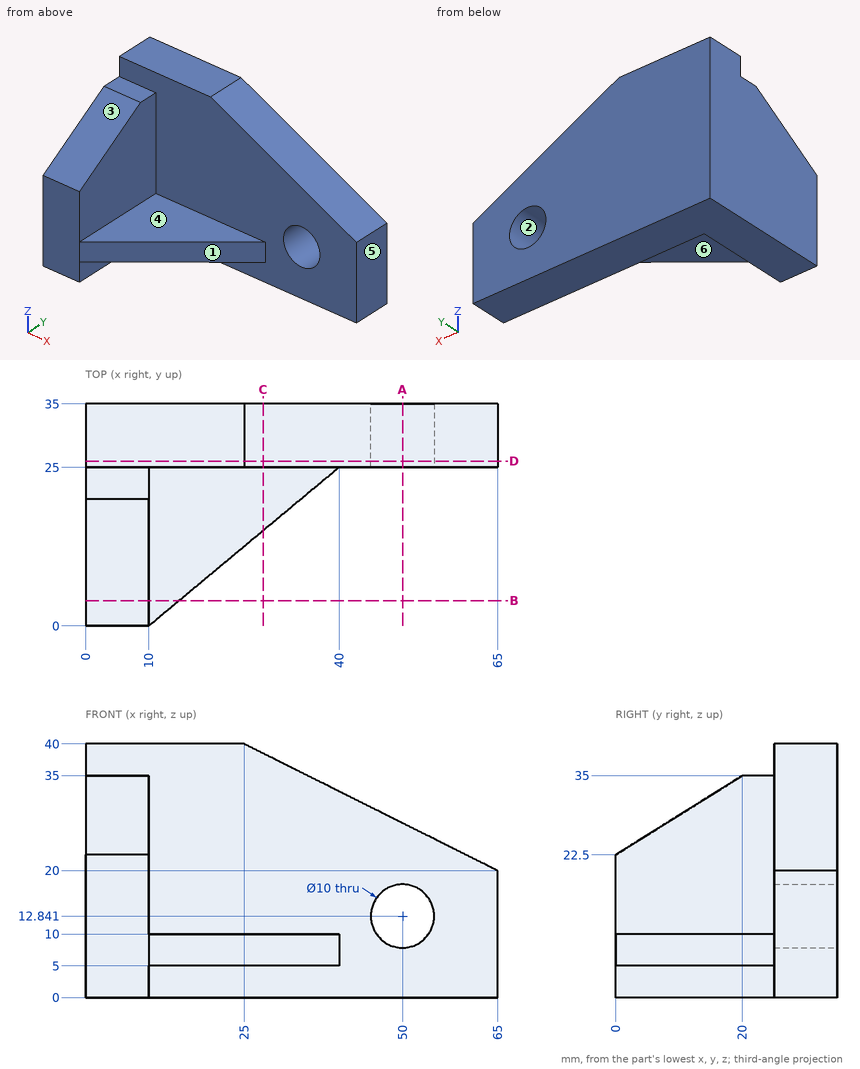
Can you work these out from the drawing? Everything is in mm from the part's minimum corner. A direction names the side the tool comes from. Coordinates: 2 decimals unless noted, no trailing zeros. Write each loop counter-clockwise with the first axis right and the second up, starting at its lowest first coordinate (ties: lowest second). Pieces come first, ordered by that corner, then holes. Notation, with made-up numbers: (23.25, 50.5) -> (71.25, 50.5) arc R28 cw to (71.25, 81.5) -> close; hole circle Ø4 at (-16.5, -7). An arc over 180 degrees is marked (long way). Write each question's results on one line, items separated by ' | '. Start each with the question number.
Item 1: If we section it at D-D, the plane y = 26: Write out the boundary of the cut face in (x, z), and give its area (3 significant figures).
Item 2: I'm going to push flat-ended pins straight in: P1, Ø4, axis at x = 18.5, y = 4, coming from the +Z side; P2, Ø7.5, axis at y = 17.5, z = 20, coming from the +X side; P3, Ø6, axis at x = 37.5, y = 19.5, coming from the +Z side; P4, Ø5.5, axis at x = 6, y = 22, coming from the +Z side. Where does each tip first touch, or does it pass through?
Item 3: Thinking about a two-plate mould opening in X: for the marked faces 1, 2 and 3, which applies, released by +X, released by -X, zero draft, split by the parting line, or undercut?
Item 4: Please list where these lines run through material, in increasing order: probe 1 along Y at (x, z) = (44.5, 8); probe 2 along X at (y, z) = (3.5, 19); probe 3 along Z at (x, y) = (50, 27).
Item 5: If we section it at B-B, the plane y = 4: Write out the boundary of the cut face in (x, z), and give its area (3 significant figures).
Item 6: If we section it at C-C, the plane x = 28: Write out the boundary of the cut face in (y, z).
Item 7: If we section it at A-A, the plane x = 50: Write out the boundary of the cut face in (y, z).
Item 8: On a 3-axis mill with a long thin cutter (end or side, diameter ignored), from which of +Z, -Z, +X, -X, +Y, -Y can I reach the whole of each face in a straight line? I mean the marked faces 4, 5 and 6. Say none if no direction works.
Answer block:
1) outline: (0, 0) -> (65, 0) -> (65, 20) -> (25, 40) -> (0, 40) -> close; hole circle Ø10 at (50, 12.84) | area: 2,120 mm²
2) P1: through | P2: x = 10 | P3: z = 10 | P4: z = 35
3) face 1: released by +X | face 2: undercut | face 3: zero draft
4) probe 1: 25 to 35 | probe 2: 0 to 10 | probe 3: 0 to 7.84, 17.84 to 27.5
5) outline: (0, 0) -> (10, 0) -> (10, 5) -> (14.8, 5) -> (14.8, 10) -> (10, 10) -> (10, 25) -> (0, 25) -> close | area: 274 mm²
6) outline: (15, 5) -> (25, 5) -> (25, 0) -> (35, 0) -> (35, 38.5) -> (25, 38.5) -> (25, 10) -> (15, 10) -> close
7) outline: (25, 0) -> (35, 0) -> (35, 7.84) -> (25, 7.84) -> close; (25, 17.84) -> (35, 17.84) -> (35, 27.5) -> (25, 27.5) -> close
8) face 4: +Z, +X, -Y | face 5: +Z, -Z, +X, +Y, -Y | face 6: -Z, +X, -Y
